Here's the drawing with two shaded views (mm, measured from the low corner). I have some questions. A direction names the side the tool comes from. Round coordinates to 2 decimals unless told otherwise and drop trailing zeros. Loops run counter-clockwise (first coordinate to the right, second up) from the corner with the lowest first, then second, coordinate; pieces in that order, holes last.
(1) Which directions (+Z, -Z, +X, -X, +Y, -Y) give clear straight access to the entire face, cutting with the end or side of a thin tool? Please do the marked faces 1 and 2.
(2) I want a section at A-A on z = 73. Write out the boundary of the cut face in (x, y) (3 decimals), plus the area to 3 significant figures.
(3) Will these pins go through, and if not, where does the flat tip stop? pin 1 Ø1.8 at (y, z) = (51, 43) entering from +X; pin 2 Ø10 at (y, z) = (59.5, 55.5) entering from +X; pin 3 Ø3 at (x, z) = (45, 44) entering from +Y.
(4) If I drill on line 1 along Z through (x, y) = (71, 56.5); line 2 along Y through (x, z) = (32, 9.5); line 3 along Z through (x, y) = (22.5, 7), over which ranges is the centre line in solid material (lowest first)?
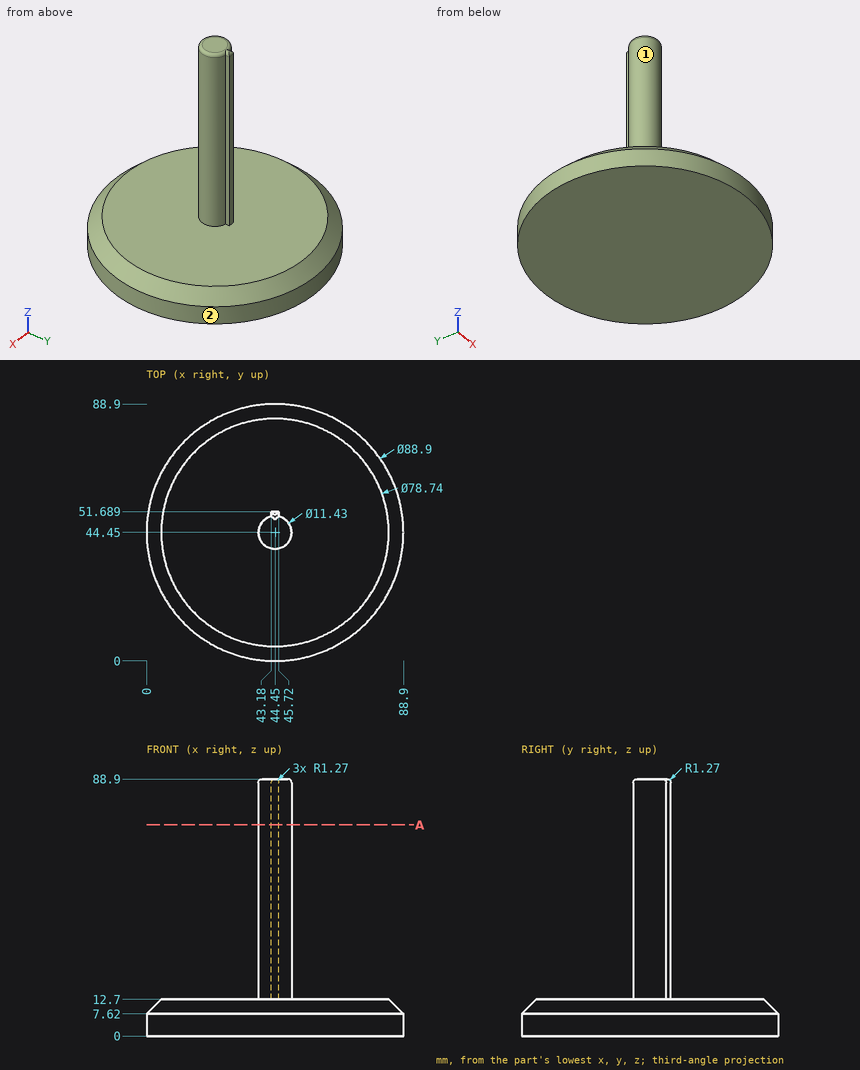
Filled sheet:
1. face 1: +Z
1. face 2: +Z, -Z
2. outline: (43.18, 50.022) arc R5.715 ccw (long way) to (45.72, 50.022) - (45.72, 51.689) - (43.18, 51.689) - close
2. area: 107 mm2
3. pin 1: stops at x = 45.72
3. pin 2: passes through
3. pin 3: stops at y = 51.69
4. line 1: z = 0 to 12.7
4. line 2: y = 3.74 to 85.16
4. line 3: z = 0 to 8.66
